Build history of the part. All positions in model axes, mm. Give positions to 0.01 mm unless a question says otherwise; leave off trailing zeros. Order: outer loops, then holes, each group sorted by start corner. A loop starts at its lowest first (then second) coordinate and runs counter-clockwise, first axis right, second up. Notation, with made-up numbers: (8, 39.5) - (65, 39.5) arc R28 cw to (65, 75.5) - close; hole circle Ø4 at (-4, 30.25). An arc over 180 degrees is marked (long way). Use a Markdown table: item, result. Add a question column.
(1) Slice it at B-B (z = 2.3). Count the separate pieces of the cut face and the enclosed holes in it, then the cut area to 3 significant figures.
(2) Wall check: line 1 (Y direction, x = -19.5, z = 1.8); line 2 (Y direction, x = -55.5, z = 3.85). Give the ranges that are in metal, low to high.
(3) Mould opens along Y. For faces 1 (the face through (-1.28, -17.814, 2.028)), 2 (the face through (-1, 2, 0)), 3 (the face through (-19.78, -17.814, 2.028)), 4 (the face through (59.02, 34.53, 1.97)) say: +Y half, -Y half, draft (parallel to the pull), parting line (faces both ways), or undercut.
(4) Slice it at A-A (x = -1). Write the cut outline in (y, z).
(5) Slice it at C-C (x = 33). Write the cut outline in (y, z), then the cut area to 3 significant figures.
from build123d import *

# Parameters (mm, degrees)
EXTRUDE_1_DEPTH     = 4
SKETCH_2_R          = 2.15
SKETCH_2_R_2        = 1.8
CUT_EXTRUDE_1_DEPTH = 4
SKETCH_3_R          = 1.682371235
SKETCH_3_R_2        = 1.63184694
SKETCH_3_R_3        = 1.6
CUT_EXTRUDE_2_DEPTH = 4


with BuildPart() as part:
    # Эскиз1 → Бобышка-Вытянуть1 (new body)
    with BuildSketch(Plane.XY):
        with BuildLine():
            Line((63, -22.965754466), (63, 25.873855155))
            ThreePointArc((63, 25.873855155), (58.922335459, 34.626385804), (50.169804811, 38.704050345))
            Line((50.169804811, 38.704050345), (-50.169804811, 38.704050345))
            ThreePointArc((-50.169804811, 38.704050345), (-58.922335459, 34.626385804), (-63, 25.873855155))
            Line((-63, 25.873855155), (-63, -22.965754466))
            ThreePointArc((-63, -22.965754466), (-58.922335459, -31.718285114), (-50.169804811, -35.795949655))
            Line((-50.169804811, -35.795949655), (50.169804811, -35.795949655))
            ThreePointArc((50.169804811, -35.795949655), (58.922335459, -31.718285114), (63, -22.965754466))
        make_face()
    extrude(amount=EXTRUDE_1_DEPTH)

    # Эскиз2 → Вырез-Вытянуть1 (cut)
    with BuildSketch(Plane.XY.offset(4)):
        with Locations((-38, -19.945949655)):
            Circle(SKETCH_2_R)
        with Locations((32.554227521, -19.442510909)):
            Circle(SKETCH_2_R_2)
        with Locations((-19.5, -19.945949655)):
            Circle(SKETCH_2_R)
        with Locations((-1, -19.945949655)):
            Circle(SKETCH_2_R)
    extrude(amount=-CUT_EXTRUDE_1_DEPTH, mode=Mode.SUBTRACT)

    # Эскиз3 → Вырез-Вытянуть2 (cut)
    with BuildSketch(Plane(origin=(0, 0, 0), x_dir=(-1, 0, 0), z_dir=(0, 0, -1))):
        with Locations((-55.991619652, 31.455233256)):
            Circle(SKETCH_3_R)
        with Locations((55.90524563, 31.455233256)):
            Circle(SKETCH_3_R_2)
        with Locations((-55.91502671, -28.516824843)):
            Circle(SKETCH_3_R_3)
        with Locations((55.91502671, -28.516824843)):
            Circle(SKETCH_3_R_3)
    extrude(amount=-CUT_EXTRUDE_2_DEPTH, mode=Mode.SUBTRACT)


solid = part.part
Solution:
| question | item | result |
|---|---|---|
| 1 | separate pieces | 1 |
| 1 | enclosed holes | 8 |
| 1 | area | 9,130 mm2 |
| 2 | line 1 | -35.8 to -22.1, -17.8 to 38.7 |
| 2 | line 2 | -34.24 to -30.06, -26.97 to 29.87, 33.04 to 37.14 |
| 3 | face 1 | undercut |
| 3 | face 2 | draft |
| 3 | face 3 | undercut |
| 3 | face 4 | +Y half |
| 4 | outline | (-35.8, 0) - (-22.1, 0) - (-22.1, 4) - (-35.8, 4) - close; (-17.8, 0) - (38.7, 0) - (38.7, 4) - (-17.8, 4) - close |
| 5 | outline | (-35.8, 0) - (-21.19, 0) - (-21.19, 4) - (-35.8, 4) - close; (-17.7, 0) - (38.7, 0) - (38.7, 4) - (-17.7, 4) - close |
| 5 | area | 284 mm2 |
